Design review of the part built by this model. Coordinates are the model's own, in mm. A direction names the side the tool comes from. Coordinates: 2 decimals unless noted, no trailing zeros. Loops run counter-clockwise (first coordinate to the right, second up) from the corner with the lowest first, then second, coordinate; pieces in that order, holes last. Notation, with made-up numbers: M 75,72 L 98,72 A18 ccw 98,90 Z; hole C 81.5,84 d8. An arc over 180 degrees is marked long. Answer as a JSON object with one key per item and string values. Group by question number.
1. Draft analysis for pull direction Z (two halves, no side actions). For faces 6 (the flat face through (-31, 43, 53)), 7 (the flat face through (-42, 24, 27)), state which applies: +Z half, -Z half, draft (parallel to the pull), parting line (faces both ways), or undercut.
2. Insertion check: pin 1 (19 mm diameter, centred on y = 45, z = 37, fed in from +X); pin 2 (4.5 mm diameter, centred on y = 34.5, z = 52, fed in from +X); pin 3 (5 mm diameter, centred on x = -10.5, z = 30.5, fed in from +Y). Each pin has a flat end and moves straight along its axis. Give the tip position at first contact, or say it passes through.
3. Consider section B-B (z = 19). State the section outline as (x, y) points, then the cut area to 3 significant figures.
4. Machinability: for faces 1 (the flat face through (-13.84, 38, 1)), 2 (the flat face through (-24, 19, 27)), 3 (the flat face through (-39, -2, 27)), 4 (the flat face through (-28, 43, 49)), 5 (the flat face through (-33.84, 43, 28)), which of the approach directions +Z, -Z, +X, -X, +Y, -Y give a long, thin tool a straight path to every point of the face, cutting with its end or side? Answer none if there is none.
5. To check wall thickness, follow probe 1 along X at (y, z) = (52.5, 5); probe 2 along X at (y, z) = (3, 50.5); probe 3 along Y at (x, z) = (-10.5, 15.5). State the ranges of each line that lie inside material, in increasing order.
6. Consider section D-D (x = -22). State the section outline as (y, z) points, then the cut area to 3 significant figures.
7. Consider section A-A (x = -7.5). State the section outline as (y, z) points.
8. Consider section C-C (y = 32.5). State the section outline as (x, z) points.
from build123d import *

# Parameters (mm, degrees)
F0_W     = 4
F0_H     = 19
F0_W_2   = 3
F1_DEPTH = 55
F2_W     = 2
F2_H     = 4
F3_DEPTH = 38
F4_SIZE  = 9
F5_SIZE  = 1


with BuildPart() as f1:
    # F0 (on Top) → F1 (new body)
    with BuildSketch(Plane.XY):
        Polygon((-0.840026, 24), (-46.840026, 24), (-46.840026, 19), (-42.840026, 19), (-3.840026, 19), (-0.840026, 19), align=None)
        with Locations((-44.840026, 9.5)):
            Rectangle(F0_W, F0_H)
        with Locations((-2.340026, 9.5)):
            Rectangle(F0_W_2, F0_H)
        Polygon((-42.840026, 0), (-46.840026, 0), (-46.840026, -2), (-31.840026, -2), (-31.840026, 0), align=None)
        Polygon((-0.840026, -2), (-0.840026, 0), (-3.840026, 0), (-20.840026, 0), (-20.840026, -2), align=None)
    extrude(amount=F1_DEPTH)

    # F2 (on face) → F3 (join)
    with BuildSketch(Plane(origin=(0, 24, 0), x_dir=(-1, 0, 0), z_dir=(0, 1, 0))):
        Polygon((36.840026, 55), (33.840026, 55), (33.840026, 53), (33.840026, 2), (33.840026, 0), (36.840026, 0), align=None)
        Polygon((33.840026, 53), (33.840026, 55), (13.840026, 55), (13.840026, 53), (23.540026, 53), (25.540026, 53), (26.840026, 53), (28.840026, 53), align=None)
        Polygon((33.840026, 0), (33.840026, 2), (28.840026, 2), (26.840026, 2), (25.540026, 2), (23.540026, 2), (13.840026, 2), (13.840026, 0), align=None)
        with Locations((27.840026, 51)):
            Rectangle(F2_W, F2_H)
        with Locations((27.840026, 4)):
            Rectangle(F2_W, F2_H)
        with Locations((24.540026, 51)):
            Rectangle(F2_W, F2_H)
        with Locations((24.540026, 4)):
            Rectangle(F2_W, F2_H)
    extrude(amount=F3_DEPTH)

    # F4
    f4_edges = [f1.edges().sort_by_distance(p)[0] for p in [
        (-13.840026, 62, 54),
        (-13.840026, 62, 1),
    ]]
    chamfer(f4_edges, length=F4_SIZE)

    # F5
    f5_edges = [f1.edges().sort_by_distance(p)[0] for p in [
        (-0.840026, -2, 27.5),
        (-46.840026, -2, 27.5),
    ]]
    chamfer(f5_edges, length=F5_SIZE)


solid = f1.part
Findings below:
{
 "1": {"face 6": "undercut", "face 7": "draft"},
 "2": {"pin 1": "stops at x = -33.84", "pin 2": "stops at x = -13.84", "pin 3": "stops at y = 24"},
 "3": {"outline": "M -46.84,-1 L -45.84,-2 L -31.84,-2 L -31.84,0 L -42.84,0 L -42.84,19 L -3.84,19 L -3.84,0 L -20.84,0 L -20.84,-2 L -1.84,-2 L -0.84,-1 L -0.84,24 L -33.84,24 L -33.84,62 L -36.84,62 L -36.84,24 L -46.84,24 Z", "area": "546 mm^2"},
 "4": {"face 1": "+Z, -Z, +X, +Y", "face 2": "+Z, -Z", "face 3": "+Z, -Z, +X, -X, -Y", "face 4": "+X, +Y", "face 5": "+Y"},
 "5": {"probe 1": "x = -36.84 to -33.84, -28.84 to -26.84, -25.54 to -23.54", "probe 2": "x = -46.84 to -42.84, -3.84 to -0.84", "probe 3": "y = -2 to 0, 19 to 24"},
 "6": {"outline": "M 19,0 L 61.16,0 L 61.16,2 L 24,2 L 24,53 L 61.16,53 L 61.16,55 L 19,55 Z", "area": "424 mm^2"},
 "7": {"outline": "M -2,0 L 0,0 L 0,55 L -2,55 Z; M 19,0 L 24,0 L 24,55 L 19,55 Z"},
 "8": {"outline": "M -36.84,0 L -13.84,0 L -13.84,2 L -23.54,2 L -23.54,6 L -25.54,6 L -25.54,2 L -26.84,2 L -26.84,6 L -28.84,6 L -28.84,2 L -33.84,2 L -33.84,53 L -28.84,53 L -28.84,49 L -26.84,49 L -26.84,53 L -25.54,53 L -25.54,49 L -23.54,49 L -23.54,53 L -13.84,53 L -13.84,55 L -36.84,55 Z"}
}
